```python
from build123d import *

# Parameters (mm, degrees)
PAD_DEPTH    = 2
SKETCH001_R  = 3.5
PAD001_DEPTH = 2
SKETCH003_R  = 1.4
PAD003_DEPTH = 2
PAD004_DEPTH = 4
FILLET_R     = 3
FILLET001_R  = 3
FILLET002_R  = 3
FILLET003_R  = 3
FILLET004_R  = 3
FILLET005_R  = 3
FILLET006_R  = 3
FILLET007_R  = 3


with BuildPart() as body:
    # Sketch → Pad (new body)
    with BuildSketch(Plane.XY):
        with BuildLine():
            Line((-36, 62.5), (36, 62.5))
            ThreePointArc((41, 57.5), (39.535534, 61.035534), (36, 62.5))
            Line((41, 57.5), (41, -57.5))
            ThreePointArc((36, -62.5), (39.535534, -61.035534), (41, -57.5))
            Line((36, -62.5), (-36, -62.5))
            ThreePointArc((-41, -57.5), (-39.535534, -61.035534), (-36, -62.5))
            Line((-41, -57.5), (-41, 57.5))
            ThreePointArc((-36, 62.5), (-39.535534, 61.035534), (-41, 57.5))
        make_face()
        with BuildLine():
            ThreePointArc((-30, 54.5), (-32.12132, 53.62132), (-33, 51.5))
            Line((-33, 39), (-33, 51.5))
            ThreePointArc((-33, 39), (-32.12132, 36.87868), (-30, 36))
            Line((30, 36), (-30, 36))
            ThreePointArc((30, 36), (32.12132, 36.87868), (33, 39))
            Line((33, 51.5), (33, 39))
            ThreePointArc((33, 51.5), (32.12132, 53.62132), (30, 54.5))
            Line((-30, 54.5), (30, 54.5))
        make_face(mode=Mode.SUBTRACT)
        with BuildLine():
            ThreePointArc((-30, -28), (-32.12132, -28.87868), (-33, -31))
            Line((-33, -51.5), (-33, -31))
            ThreePointArc((-33, -51.5), (-32.12132, -53.62132), (-30, -54.5))
            Line((30, -54.5), (-30, -54.5))
            ThreePointArc((30, -54.5), (32.12132, -53.62132), (33, -51.5))
            Line((33, -31), (33, -51.5))
            ThreePointArc((33, -31), (32.12132, -28.87868), (30, -28))
            Line((-30, -28), (30, -28))
        make_face(mode=Mode.SUBTRACT)
        with BuildLine():
            ThreePointArc((-30, 22), (-32.12132, 21.12132), (-33, 19))
            Line((-33, -11), (-33, 19))
            ThreePointArc((-33, -11), (-32.12132, -13.12132), (-30, -14))
            Line((30, -14), (-30, -14))
            ThreePointArc((30, -14), (32.12132, -13.12132), (33, -11))
            Line((33, 19), (33, -11))
            ThreePointArc((33, 19), (32.12132, 21.12132), (30, 22))
            Line((-30, 22), (30, 22))
        make_face(mode=Mode.SUBTRACT)
    extrude(amount=PAD_DEPTH)

    # Sketch001 → Pad001 (join)
    with BuildSketch(Plane(origin=(7.5, -20, 0), x_dir=(1, 0, 0), z_dir=(0, -1, 0))):
        with BuildLine():
            Line((10.4, 27), (10.4, 6))
            Line((33.5, 6), (10.4, 6))
            Line((33.5, 2), (33.5, 6))
            Line((-48.5, 2), (33.5, 2))
            Line((-48.5, 6), (-48.5, 2))
            Line((-25.4, 6), (-48.5, 6))
            Line((-25.4, 6), (-8.817564, 32.514577))
            ThreePointArc((10.4, 27), (2.868565, 36.996566), (-8.817564, 32.514577))
        make_face()
        with Locations((0, 27)):
            Circle(SKETCH001_R, mode=Mode.SUBTRACT)
    extrude(amount=PAD001_DEPTH)

    # Sketch003 → Pad003 (join)
    with BuildSketch(Plane(origin=(7.5, 30, 0), x_dir=(1, 0, 0), z_dir=(0, -1, 0))):
        with BuildLine():
            Line((33.5, 2), (-48.5, 2))
            Line((-48.5, 6), (-48.5, 2))
            Line((-25.4, 6), (-48.5, 6))
            Line((-8.817564, 32.514577), (-25.4, 6))
            ThreePointArc((10.4, 27), (2.868565, 36.996566), (-8.817564, 32.514577))
            Line((10.4, 27), (10.4, 6))
            Line((10.4, 6), (33.5, 6))
            Line((33.5, 6), (33.5, 2))
        make_face()
        with Locations((0, 27)):
            Circle(SKETCH003_R, mode=Mode.SUBTRACT)
        with Locations((-7, 27)):
            Circle(SKETCH003_R, mode=Mode.SUBTRACT)
        with Locations((0, 20)):
            Circle(SKETCH003_R, mode=Mode.SUBTRACT)
        with Locations((7, 27)):
            Circle(SKETCH003_R, mode=Mode.SUBTRACT)
        with Locations((0, 34)):
            Circle(SKETCH003_R, mode=Mode.SUBTRACT)
    extrude(amount=PAD003_DEPTH)

    # Sketch004 (on Face5 of Pad003) → Pad004 (join)
    with BuildSketch(Plane.XY.offset(2)):
        with BuildLine():
            Line((-36, 62.5), (36, 62.5))
            ThreePointArc((41, 57.5), (39.535534, 61.035534), (36, 62.5))
            Line((41, -57.5), (41, 57.5))
            ThreePointArc((36, -62.5), (39.535534, -61.035534), (41, -57.5))
            Line((-36, -62.5), (36, -62.5))
            ThreePointArc((-41, -57.5), (-39.535534, -61.035534), (-36, -62.5))
            Line((-41, 57.5), (-41, -57.5))
            ThreePointArc((-36, 62.5), (-39.535534, 61.035534), (-41, 57.5))
        make_face()
        with BuildLine():
            Line((-36, 60.5), (36, 60.5))
            ThreePointArc((39, 57.5), (38.12132, 59.62132), (36, 60.5))
            Line((39, 57.5), (39, -57.5))
            ThreePointArc((36, -60.5), (38.12132, -59.62132), (39, -57.5))
            Line((36, -60.5), (-36, -60.5))
            ThreePointArc((-39, -57.5), (-38.12132, -59.62132), (-36, -60.5))
            Line((-39, -57.5), (-39, 57.5))
            ThreePointArc((-36, 60.5), (-38.12132, 59.62132), (-39, 57.5))
        make_face(mode=Mode.SUBTRACT)
    extrude(amount=PAD004_DEPTH)

    # Fillet
    fillet_edges = [body.edges().sort_by_distance(p)[0] for p in [
        (-39, 4, 2),
    ]]
    fillet(fillet_edges, radius=FILLET_R)

    # Fillet001
    fillet001_edges = [body.edges().sort_by_distance(p)[0] for p in [
        (-39, -39.75, 2),
    ]]
    fillet(fillet001_edges, radius=FILLET001_R)

    # Fillet002
    fillet002_edges = [body.edges().sort_by_distance(p)[0] for p in [
        (0, -22, 2),
    ]]
    fillet(fillet002_edges, radius=FILLET002_R)

    # Fillet003
    fillet003_edges = [body.edges().sort_by_distance(p)[0] for p in [
        (1.5, 28, 2),
    ]]
    fillet(fillet003_edges, radius=FILLET003_R)

    # Fillet004
    fillet004_edges = [body.edges().sort_by_distance(p)[0] for p in [
        (1.5, -20, 2),
    ]]
    fillet(fillet004_edges, radius=FILLET004_R)

    # Fillet005
    fillet005_edges = [body.edges().sort_by_distance(p)[0] for p in [
        (39, 4, 2),
    ]]
    fillet(fillet005_edges, radius=FILLET005_R)

    # Fillet006
    fillet006_edges = [body.edges().sort_by_distance(p)[0] for p in [
        (0, 60.5, 2),
    ]]
    fillet(fillet006_edges, radius=FILLET006_R)

    # Fillet007
    fillet007_edges = [body.edges().sort_by_distance(p)[0] for p in [
        (0, 30, 2),
    ]]
    fillet(fillet007_edges, radius=FILLET007_R)


with BuildPart() as part_mirroring:
    # Part__Mirroring: instance of Body
    add(body.part.mirror(Plane(origin=(0, 0, 0), x_dir=(0, -1, 0), z_dir=(1, 0, 0))))


solid = part_mirroring.part
```
Input: part model. Units: mm. Frame: model coordinates. A direction names the side the tool comes from. Coordinates: 2 decimals unless noted, no trailing zeros. Write each loop counter-clockwise with the first axis right and the second up, starting at its lowest first coordinate (ties: lowest second). Pieces come first, ordered by that corner, then holes. Notation, with made-up numbers: M -16.5,51.25 L 22.5,51.25 A30 cw 22.5,84.25 Z; hole C 38,22 d7. An arc over 180 degrees is marked long. Use one line per item in the form item = value.
Q1. First-contact query: pin 1 (9.5 mm diameter, centred on x = 6, z = 15, fed in from +Y); pin 2 (8 mm diameter, centred on x = -32.5, y = 46.5, fed in from -Z); pin 3 (3.5 mm diameter, centred on x = -7.5, z = 34, fed in from -Y); pin 4 (1.6 mm diameter, centred on y = -20.5, z = 18.5, fed in from -X). Flat tips, straight axial feed; report the tip coordinate or a pass-through.
Answer below:
pin_1 = 30
pin_2 = 0
pin_3 = -22
pin_4 = -17.9
Q2. Draft query along X for faces 1 (the face through (-38.14, 45.08, 2.9)), 2 (the face through (-1, -62.5, 3)), 3 (the face through (-10.549, 29.014, 36.943)). Return one class per face: released by +X, released by -X, zero draft, split by the parting line, or undercut.
Answer below:
face_1 = undercut
face_2 = zero draft
face_3 = split by the parting line
Q3. Set-up query: faces 4 (the face through (38.1, 4.29, 2.86)), 5 (the face through (-0.197, 29.014, 25.633)), 6 (the face through (32.14, -13.1, 0.99)). Return all of +Z, -Z, +X, -X, +Y, -Y with unobstructed straight access to the full face (end or side cutting, diameter ignored); none if empty.
Answer below:
face_4 = +Z
face_5 = +Y
face_6 = +Z, -Z
Q4. Section A-A (y = -6). Return loops of the section in (x, z), plus the area to 3 significant figures.
Answer below:
outline = M -41,0 L -33,0 L -33,2 L -36,2 A3 cw -39,5 L -39,6 L -41,6 Z; M 33,0 L 41,0 L 41,6 L 39,6 L 39,5 A3 cw 36,2 L 33,2 Z
area = 51.9 mm²
Q5. Section B-B (x = -31.5). Count the separate pieces of the cut face and the enclosed holes in it, plus the area to 3 significant figures.
Answer below:
separate_pieces = 4
enclosed_holes = 0
area = 136 mm²
Q6. Material intervals for probe 1 along Z at (x, y) = (-7.5, -21); probe 2 along Y at (x, z) = (1.5, 10); probe 3 along Z at (x, y) = (-7, 29), sorted ascending. Write a range as from..to.
Answer below:
probe_1 = 0..23.5, 30.5..37.4
probe_2 = -22..-20, 28..30
probe_3 = 0..18.69, 21.31..25.69, 28.31..32.69, 35.31..37.39
Q7. Section C-C (z = 14.5). Return loops of the section in (x, y), plus the area to 3 significant figures.
Answer below:
outline = M -17.9,-22 L 12.58,-22 L 12.58,-20 L -17.9,-20 Z; M -17.9,28 L 12.58,28 L 12.58,30 L -17.9,30 Z
area = 122 mm²
